Autodesk Inventor part; units mm, degrees
ref_plane "YZ Plane" through (0, 0, 0) normal (1, 0, 0) x (0, 1, 0)
ref_plane "XZ Plane" through (0, 0, 0) normal (0, 1, 0) x (-1, 0, 0)
ref_plane "XY Plane" through (0, 0, 0) normal (0, 0, 1) x (1, 0, 0)
sketch "Szkic1" plane through (0, 0, 0) normal (0, 1, 0) x (-1, 0, 0)
  circle A0 centre (0, 0) radius 7.75
  dimension "d0" = 15.5
extrude "Wyciągnięcie proste1" add sketch "Szkic1" along normal blind 17
hole "Otwór1" at (0, 0, 0) direction (0, 1, 0) diameter 9.728 depth 12
chamfer "Faza1" distance 0.8 angle 45 1 edges at (7.75, 17, 0)
sketch "Szkic2" plane through (0, 17, 0) normal (0, 1, 0) x (1, 0, 0)
  circle A0 centre (0, 0) radius 6.95
  line L0 (-4.5, 0) -> (4.5, 0) construction
  line L1 (-4.5, -0.875) -> (4.5, -0.875)
  line L2 (4.5, 0.875) -> (-4.5, 0.875)
  arc A1 (-4.5, 0.875) -> (-4.5, -0.875) centre (-4.5, 0) ccw
  arc A2 (4.5, -0.875) -> (4.5, 0.875) centre (4.5, 0) ccw
  point P0 (0, 0.875)
  dimension "d15" = 1.75
  dimension "d16" = 9
extrude "Wyciągnięcie proste2" cut sketch "Szkic2" against normal blind 1 contours A1 L2 A2 L1
pattern_circular "Szyk kołowy1" count 4 over 360 about axis through (0, 0, 0) along (0, 1, 0) of "Wyciągnięcie proste2"
properties part number "Filtr HOT 3P -korek" material "Tworzywo sztuczne PBT"
Input: part model. Units: mm. Frame: model coordinates. A direction names the side the tool comes from. Round coordinates to 2 decimals unless told otherwise and drop trailing zeros. Write each loop counter-clockwise with the first axis right and the second up, starting at its lowest first coordinate (ties: lowest second). Pieces come first, ordered by that corner, then holes.
1) Contact query for flat-ended pins moving along their axis: P1, Ø1.1, axis at y = 16.5, z = 2.5, coming from the +X side; P2, Ø3, axis at x = 1.5, z = 0, coming from the -Y side; P3, Ø1.1, axis at x = 3, y = 16.5, coming from the +Z side. Output: stop coordinate, or through.
2) Cut plane A-A (z = 0). Return the cut outline in (x, y) (3 decimals).
3) Cut plane B-B (y = 2.25). Return the cut outline in (x, z).
4) Ray query, L1, parallel to Z at x = 0, y = 11; L2, parallel to Y at x = 3.75, z = 1.5; L3, parallel to Z at x = -1.5, y = 1.5. Return the intervals inside material, ascending.
5) Cut plane C-C (x = 0). Return the cut outline in (y, z) (3 decimals), then the cut area to 3 significant figures.
6) Reachability of faces 4 (the flat face through (2.7, 16.5, -0.875)), 5 (the flat face through (0.1, 0, -5.1)), 6 (the cylindrical face through (-1.46, 6.08, -4.64)) from +Z, -Z, +X, -X, +Y, -Y: full face, straight path, thin tool, end or side. Return the list, or none.
7) Cut plane D-D (y = 13.75). Return the cut outline in (x, z).
8) Draft query along Z for faces 1 (the flat face through (-1.4, 17, -1.4)), 2 (the flat face through (-0.875, 16.5, -2.7)), 3 (the cylindrical face through (1.009, 7.987, -7.684)). Return one class per face: pulls with the +Z half, pulls with the -Z half, needs draft (parallel to the pull), parting line crosses it, or undercut.
Geometry says:
1. P1: stops at x = 7.48
1. P2: stops at y = 12
1. P3: stops at z = 7.32
2. outline: (-7.75, 0) - (-4.864, 0) - (-4.864, 12) - (4.864, 12) - (4.864, 0) - (7.75, 0) - (7.75, 16.2) - (6.95, 17) - (5.375, 17) - (5.375, 16) - (-5.375, 16) - (-5.375, 17) - (-6.95, 17) - (-7.75, 16.2) - close
3. outline: circle Ø15.5 at (0, 0); hole circle Ø9.73 at (0, 0)
4. L1: z = -7.75 to -4.86, 4.86 to 7.75
4. L2: y = 12 to 17
4. L3: z = -7.6 to -4.63, 4.63 to 7.6
5. outline: (0, -7.75) - (16.2, -7.75) - (17, -6.95) - (17, -5.375) - (16, -5.375) - (16, 5.375) - (17, 5.375) - (17, 6.95) - (16.2, 7.75) - (0, 7.75) - (0, 4.864) - (12, 4.864) - (12, -4.864) - (0, -4.864) - close
5. area: 135 mm2
6. face 4: +Y
6. face 5: +Z, -Z, +X, -X, -Y
6. face 6: -Y
7. outline: circle Ø15.5 at (0, 0)
8. face 1: needs draft
8. face 2: undercut
8. face 3: parting line crosses it
